CAD build for the part. Positions are in the model's coordinates, mm. A direction names the side the tool comes from. Give positions to 0.01 mm unless a question says otherwise; leave off trailing zeros. Loops run counter-clockwise (first coordinate to the right, second up) from the corner with the lowest first, then second, coordinate; pieces in that order, holes last.
```python
from build123d import *

# Parameters (mm, degrees)
F0_W        = 47.4317967892
F0_H        = 20
F0_R        = 4.5
F1_DEPTH    = 15
F2_R        = 7.05
F3_DEPTH    = 25
F7_DEPTH    = 13.25
F8_T1_DEPTH = 20
F9_START    = 10
F0_R_2      = 2.5
F9_DEPTH    = 5


# Not quite as in the source:
# - a fillet or chamfer that OpenCascade refuses, or shapes differently, is made with other operations: its cross-section is extruded or revolved along the edge and cut away or added


with BuildPart() as f1:
    # F0 (on Front) → F1 (new body)
    with BuildSketch(Plane.XZ):
        Rectangle(F0_W, F0_H)
        with Locations((-18.2158983946, 0)):
            Circle(F0_R, mode=Mode.SUBTRACT)
        with Locations((18.2158983946, 0)):
            Circle(F0_R, mode=Mode.SUBTRACT)
    extrude(amount=F1_DEPTH)

    # F2 (on face) → F3 (cut)
    with BuildSketch(Plane.XY.offset(10)):
        with Locations((0, -15)):
            Circle(F2_R)
    extrude(amount=-F3_DEPTH, mode=Mode.SUBTRACT)

    # F4 (on face) → F5 (revolve, cut)
    with BuildSketch(Plane.XZ.offset(15)):
        with BuildLine():
            Line((-7.05, -10), (-7.05, 10))
            ThreePointArc((-7.05, 10), (-12.2352972992, 0), (-7.05, -10))
        make_face()
    revolve(axis=Axis((0, -15, 0.0368109904), (0, 0, -1)), mode=Mode.SUBTRACT)

    # F6 (on face) → F7 (cut)
    with BuildSketch(Plane.XZ.offset(15)):
        Polygon((2.5, -10.0813228637), (2.5, 10), (0, 10), (-2.5, 10), (-2.5, -10.0813228637), (0, -10.0813228637), align=None)
    extrude(amount=-F7_DEPTH, mode=Mode.SUBTRACT)

    # F8: fillet of radius 1 on 2 edges, made by hand

    # F8_s2 → F8_t1 (join)
    with BuildSketch(Plane.XY.offset(-10)):
        with BuildLine():
            add(Edge.make_bspline(
                [(1.5, -1.75), (2.5, -1.75), (2.5, -2.75)],
                knots=[0, 0, 0, 1, 1, 1], degree=2, weights=[1, 2.3333333333, 1]))
            Line((2.5, -2.75), (2.5, -1.75))
            Line((2.5, -1.75), (1.5, -1.75))
        make_face()
        with BuildLine():
            add(Edge.make_bspline(
                [(-2.5, -2.75), (-2.5, -1.75), (-1.5, -1.75)],
                knots=[0, 0, 0, 1, 1, 1], degree=2, weights=[1, 2.3333333333, 1]))
            Line((-1.5, -1.75), (-2.5, -1.75))
            Line((-2.5, -1.75), (-2.5, -2.75))
        make_face()
    extrude(amount=F8_T1_DEPTH)

    # F0 (on Front) → F9 (join)
    with BuildSketch(Plane.XZ.offset(F9_START)):
        with Locations((-18.2158983946, 0)):
            Circle(F0_R)
        with Locations((-18.2158983946, 0)):
            Circle(F0_R_2, mode=Mode.SUBTRACT)
        with Locations((18.2158983946, 0)):
            Circle(F0_R)
        with Locations((18.2158983946, 0)):
            Circle(F0_R_2, mode=Mode.SUBTRACT)
    extrude(amount=F9_DEPTH)


solid = f1.part
```
1. Saw through at C-C, the plane z = 0. Count the separate pieces of the cut face and the enclosed holes in it, and give its area (3 significant figures).
Responses:
separate pieces: 3
enclosed holes: 0
area: 241 mm2
2. Drop flat-ended pins along their axis: pin 1 (4 mm diameter, centred on x = -18.22, z = 0, fed in from -Y); pin 2 (1.5 mm diameter, centred on x = 0, z = 0.5, fed in from -Y); pin 3 (8 mm diameter, centred on x = 18.22, z = 0, fed in from +Y). Give the stop position or say it passes through.
Responses:
pin 1: passes through
pin 2: stops at y = -1.75
pin 3: stops at y = -10
3. Probe line 1 along X through (y, z) = (-3, 5.5); line 2 along X through (y, z) = (-6.25, 4); line 3 along Y through (x, z) = (-1, -1.25). List the from-to ranges inside material, lowest first.
Responses:
line 1: x = -23.72 to -2.5, 2.5 to 23.72
line 2: x = -23.72 to -20.28, -16.15 to -7.56, 7.56 to 16.15, 20.28 to 23.72
line 3: y = -1.75 to 0
4. Tool access for faces 1 (the face through (22.51, -4.93, 1.35)), 2 (the face through (2.5, -3, -2)), 3 (the face through (15, -15, 0)): list every direction of +Z, -Z, +X, -X, +Y, -Y with a clear straight run to the whole face (end or side of a thin tool).
Responses:
face 1: +Y
face 2: +Z, -Z, -Y
face 3: +Z, -Z, +X, -X, -Y
5. Saw through at A-A, the plane y = -7. List the corners of the cut face in (x, z), and give its area (3 significant figures).
Responses:
outline: (-23.72, -10) - (-2.5, -10) - (-2.5, -8.91) arc R9.26 cw to (-2.5, 8.91) - (-2.5, 10) - (-23.72, 10) - close; (2.5, -10) - (23.72, -10) - (23.72, 10) - (2.5, 10) - (2.5, 8.91) arc R9.26 cw to (2.5, -8.91) - close; hole circle Ø9 at (-18.22, 0); hole circle Ø9 at (18.22, 0)
area: 544 mm2
6. Pull direction X, two halves, no side cores. Call faces 4 (the face through (23.716, -7, 0)), 5 (the face through (0, 0, 0)), 6 (the face through (-23.716, -7, 0)), 7 (the face through (0, -1.75, 0)): released by +X, released by -X, zero draft, split by the parting line, or undercut.
Responses:
face 4: released by +X
face 5: zero draft
face 6: released by -X
face 7: undercut
7. Saw through at D-D, the plane x = -15. List the corners of the cut face in (y, z).
Responses:
outline: (-15, -10) - (0, -10) - (0, -3.15) - (-10, -3.15) - (-10, 3.15) - (0, 3.15) - (0, 10) - (-15, 10) - close
8. Saw through at B-B, the plane x = 17.5. List the corners of the cut face in (y, z).
Responses:
outline: (-15, -10) - (0, -10) - (0, -4.44) - (-10, -4.44) - (-10, -2.4) - (-15, -2.4) - close; (-15, 2.4) - (-10, 2.4) - (-10, 4.44) - (0, 4.44) - (0, 10) - (-15, 10) - close
